```python
from build123d import *

# Parameters (mm, degrees)
EXTRUDE_1_DEPTH     = 40.8
SKETCH_4_W          = 41.6
SKETCH_4_H          = 29.6
CUT_EXTRUDE_1_DEPTH = 5
EXTRUDE_2_DEPTH     = 0.8
CUT_EXTRUDE_2_DEPTH = 49.380161223


with BuildPart() as part:
    # 草圖1 → 填料-伸長1 (new body)
    with BuildSketch(Plane(origin=(0, 0, 0), x_dir=(1, 0, 0), z_dir=(0, 1, 0))):
        with BuildLine():
            Line((-10, -15.6), (10, -15.6))
            ThreePointArc((10, -15.6), (17.636753237, -12.436753237), (20.8, -4.8))
            Line((20.8, -4.8), (20.8, 4.8))
            ThreePointArc((20.8, 4.8), (17.636753237, 12.436753237), (10, 15.6))
            Line((10, 15.6), (-10, 15.6))
            ThreePointArc((-10, 15.6), (-17.636753237, 12.436753237), (-20.8, 4.8))
            Line((-20.8, 4.8), (-20.8, -4.8))
            ThreePointArc((-20.8, -4.8), (-17.636753237, -12.436753237), (-10, -15.6))
        make_face()
        with BuildLine():
            Line((-10, -14.8), (10, -14.8))
            ThreePointArc((10, -14.8), (17.071067812, -11.871067812), (20, -4.8))
            Line((20, -4.8), (20, 4.8))
            ThreePointArc((20, 4.8), (17.071067812, 11.871067812), (10, 14.8))
            Line((10, 14.8), (-10, 14.8))
            ThreePointArc((-10, 14.8), (-17.071067812, 11.871067812), (-20, 4.8))
            Line((-20, 4.8), (-20, -4.8))
            ThreePointArc((-20, -4.8), (-17.071067812, -11.871067812), (-10, -14.8))
        make_face(mode=Mode.SUBTRACT)
    extrude(amount=EXTRUDE_1_DEPTH)

    # 草圖4 → 除料-伸長1 (cut)
    with BuildSketch(Plane(origin=(0, 40.8, 0), x_dir=(1, 0, 0), z_dir=(0, 1, 0))):
        Rectangle(SKETCH_4_W, SKETCH_4_H)
    extrude(amount=-CUT_EXTRUDE_1_DEPTH, mode=Mode.SUBTRACT)

    # 草圖5 → 填料-伸長2 (add)
    with BuildSketch(Plane.XZ):
        with BuildLine():
            Line((20, 4.8), (20, -4.8))
            ThreePointArc((20, -4.8), (17.071067812, -11.871067812), (10, -14.8))
            Line((10, -14.8), (-10, -14.8))
            ThreePointArc((-10, -14.8), (-17.071067812, -11.871067812), (-20, -4.8))
            Line((-20, -4.8), (-20, 4.8))
            ThreePointArc((-20, 4.8), (-17.071067812, 11.871067812), (-10, 14.8))
            Line((-10, 14.8), (10, 14.8))
            ThreePointArc((10, 14.8), (17.071067812, 11.871067812), (20, 4.8))
        make_face()
    extrude(amount=-EXTRUDE_2_DEPTH)

    # 草圖7 → 除料-伸長2 (cut, through all)
    with BuildSketch(Plane.XZ):
        with BuildLine():
            Line((-7.4, 7.1), (-7.4, -7.1))
            ThreePointArc((-7.4, -7.1), (0, -14.5), (7.4, -7.1))
            Line((7.4, -7.1), (7.4, 7.1))
            ThreePointArc((7.4, 7.1), (0, 14.5), (-7.4, 7.1))
        make_face()
    extrude(amount=-CUT_EXTRUDE_2_DEPTH, mode=Mode.SUBTRACT)


solid = part.part
```
For this review, take the finished solid that the model builds, in its own axes (mm). A direction names the side the tool comes from. Round coordinates to 2 decimals unless told otherwise and drop trailing zeros. Loops run counter-clockwise (first coordinate to the right, second up) from the corner with the lowest first, then second, coordinate; pieces in that order, holes last.
Q1. Insertion check: pin 1 Ø3 at (x, z) = (-13.5, -2) entering from +Y; pin 2 Ø12 at (x, z) = (-15, 0.5) entering from +Y; pin 3 Ø1.5 at (x, z) = (5.5, -3.5) entering from +Y. Each pin has a flat end and moves straight along its axis. Give the tip position at first contact, or say it passes through.
Result sheet:
pin 1: stops at y = 0.8
pin 2: stops at y = 35.8
pin 3: passes through
Q2. Add section B-B on z = 10.5. Write out the cut boundary in (x, y), plus the area to 3 significant figures.
Result sheet:
outline: (-19.17, 0) - (-6.57, 0) - (-6.57, 0.8) - (-18.22, 0.8) - (-18.22, 35.8) - (-19.17, 35.8) - close; (6.57, 0) - (19.17, 0) - (19.17, 35.8) - (18.22, 35.8) - (18.22, 0.8) - (6.57, 0.8) - close
area: 87.1 mm2
Q3. Machinability: for faces 4 (the face through (-20.8, 18, 0)), 5 (the face through (0.16, 0.39, 14.5)), 6 (the face through (-16.99, 18.05, -11.95)), which of the approach directions +Z, -Z, +X, -X, +Y, -Y give a long, thin tool a straight path to every point of the face, cutting with its end or side? Answer none if there is none.
Result sheet:
face 4: +Z, -Z, -X, +Y, -Y
face 5: +Y, -Y
face 6: +Y
Q4. Add section D-D on x = -17. Write out the cut boundary in (y, z), plus the area to 3 significant figures.
Result sheet:
outline: (0, -13.02) - (35.8, -13.02) - (35.8, -11.94) - (0.8, -11.94) - (0.8, 11.94) - (35.8, 11.94) - (35.8, 13.02) - (0, 13.02) - close
area: 96.6 mm2
Q5. Add section C-C on y = 29. Write out the cut boundary in (x, z).
Result sheet:
outline: (-20.8, -4.8) arc R10.8 ccw to (-10, -15.6) - (10, -15.6) arc R10.8 ccw to (20.8, -4.8) - (20.8, 4.8) arc R10.8 ccw to (10, 15.6) - (-10, 15.6) arc R10.8 ccw to (-20.8, 4.8) - close; hole (-20, -4.8) arc R10 ccw to (-10, -14.8) - (10, -14.8) arc R10 ccw to (20, -4.8) - (20, 4.8) arc R10 ccw to (10, 14.8) - (-10, 14.8) arc R10 ccw to (-20, 4.8) - close
Q6. To check wall thickness, follow line 1 along X through (y, z) = (33.5, 2); line 2 along Z through (x, y) = (3, 12); line 3 along Y through (x, z) = (14, 14). State the ranges of each line that lie inside material, in increasing order.
Result sheet:
line 1: x = -20.8 to -20, 20 to 20.8
line 2: z = -15.6 to -14.8, 14.8 to 15.6
line 3: y = 0 to 35.8
Q7. Mouldability with a two-part tool opening along Z and no side actions: class faces 1 (the face through (0, 20, 15.6)), 2 (the face through (10, 0, 0)), 3 (the face through (17.15, 18.05, -11.79)) as +Z half, -Z half, draft (parallel to the pull), parting line (faces both ways), or undercut.
Result sheet:
face 1: +Z half
face 2: draft
face 3: undercut
Q8. Add section A-A on x = 0. Write out the cut boundary in (y, z), plus the area to 3 significant figures.
Result sheet:
outline: (0, -15.6) - (40.8, -15.6) - (40.8, -14.8) - (0.8, -14.8) - (0.8, -14.5) - (0, -14.5) - close; (0, 14.5) - (0.8, 14.5) - (0.8, 14.8) - (40.8, 14.8) - (40.8, 15.6) - (0, 15.6) - close
area: 65.8 mm2
